Print and shaded views of the part. All mm, measured from the part's lowest x, y and z. A direction names the side the tool comes from. Coordinates: 2 decimals unless noted, no trailing zeros. Order: outer loops, then holes, each group sorted by start corner. A loop starts at its lowest first (then second) coordinate and runs counter-clockwise, first axis right, second up.
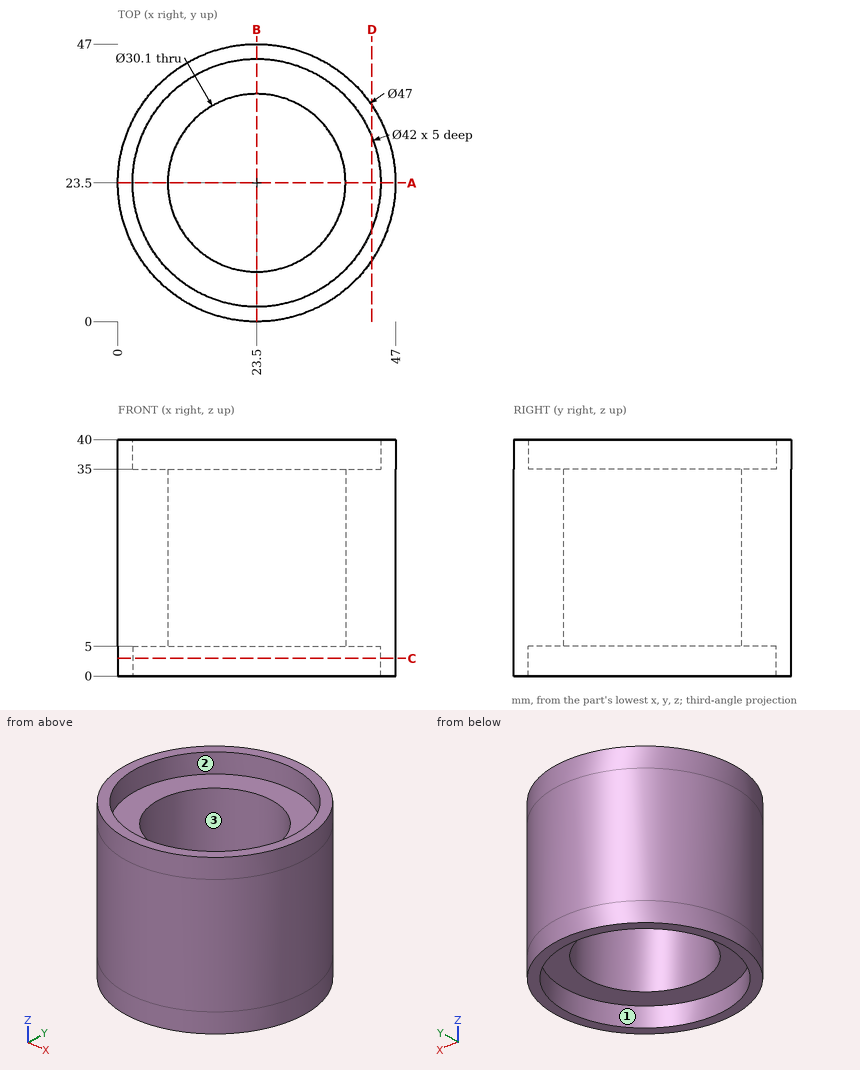
Q1. Cut at A-A, the plane y = 23.5. List the corners of the cut face in (x, z).
Established:
outline: (0, 0) - (2.5, 0) - (2.5, 5) - (8.45, 5) - (8.45, 35) - (2.5, 35) - (2.5, 40) - (0, 40) - close; (38.55, 5) - (44.5, 5) - (44.5, 0) - (47, 0) - (47, 40) - (44.5, 40) - (44.5, 35) - (38.55, 35) - close
Q2. Cut at C-C, the plane z = 3. List the corners of the cut face in (x, y).
Established:
outline: circle Ø47 at (23.5, 23.5); hole circle Ø42 at (23.5, 23.5)
Q3. Probe line 1 (Y direction, x = 23, z = 20); line 2 (Y direction, x = 23, z = 38). List the from-to ranges inside material, lowest first.
Established:
line 1: y = 0.01 to 8.46, 38.54 to 46.99
line 2: y = 0.01 to 2.51, 44.49 to 46.99
Q4. Drop flat-ended pins along their axis: P1, Ø10, axis at x = 37, z = 25, coming from the -Y side; P2, Ø12, axis at y = 9, z = 18, coming from the -X side; P3, Ø1.5, axis at x = 14.5, y = 14.5, coming from the -Z side; P4, Ø1.5, axis at y = 35.5, z = 19, coming from the +X side. Give the stop position or say it passes through.
Established:
P1: stops at y = 1.59
P2: stops at x = 1.59
P3: passes through
P4: stops at x = 44.13
Q5. Cut at D-D, the plane x = 43. List the corners of the cut face in (y, z), plus the area to 3 significant figures.
Established:
outline: (10.39, 0) - (15.71, 0) - (15.71, 5) - (31.29, 5) - (31.29, 0) - (36.61, 0) - (36.61, 40) - (31.29, 40) - (31.29, 35) - (15.71, 35) - (15.71, 40) - (10.39, 40) - close
area: 893 mm2
Q6. Which spindle directions (+Z, -Z, +X, -X, +Y, -Y) get a long thin tool onto all of the face, cutting with end or side? Do the marked faces 1, 2 and 3. Say none if no direction does.
Established:
face 1: -Z
face 2: +Z
face 3: +Z, -Z
